For this review, take the finished solid that the model builds, in its own axes (mm). Face numbers are marked on the shaded views. A direction names the side the tool comes from. Round coordinates to 2 decimals unless told otherwise and drop trailing zeros. Write each loop counter-clockwise with the first axis right and the second up, starting at its lowest first coordinate (ties: lowest second). Pieces come first, ordered by that corner, then holes.
from build123d import *

# Parameters (mm, degrees)
SWEEP_THIN1_PROFILE_R   = 10
SWEEP_THIN1_PROFILE_R_2 = 7
SKETCH22_R              = 5
CUT_EXTRUDE1_DEPTH      = 542.256514583
CUT_EXTRUDE1_DEPTH_BACK = 542.256514583


with BuildPart() as part:
    # Sweep-Thin1: sweep along a path in Sketch1
    with BuildLine(Plane(origin=(0, 0, 0), x_dir=(1, 0, 0), z_dir=(0, 1, 0))) as sweep_thin1_path:
        Line((0, 0), (-169.705627485, 169.705627485))
        ThreePointArc((-169.705627485, 169.705627485), (-185.926794926, 180.544265051), (-205.060966544, 184.350288425))
        Line((-205.060966544, 184.350288425), (-505.060966544, 184.350288425))
    # Sweep-Thin1 profile (on start of the path) → Sweep-Thin1 (sweep)
    with BuildSketch(Plane(origin=(0, 0, 0), x_dir=(-0.7071067811865487, 0, 0.7071067811865465), z_dir=(-0.7071067811865465, 0, -0.7071067811865487))):
        Circle(SWEEP_THIN1_PROFILE_R)
        Circle(SWEEP_THIN1_PROFILE_R_2, mode=Mode.SUBTRACT)
    sweep(path=sweep_thin1_path.line)

    # Sketch22 → Cut-Extrude1 (cut, two sides)
    with BuildSketch(Plane(origin=(0, 0, 0), x_dir=(1, 0, 0), z_dir=(0, 1, 0))) as cut_extrude1_sk:
        with Locations(Location((-35.355339059, 35.355339059, 0), (0, 0, 270))):
            Circle(SKETCH22_R)
    extrude(amount=CUT_EXTRUDE1_DEPTH, mode=Mode.SUBTRACT)
    extrude(cut_extrude1_sk.sketch, amount=-CUT_EXTRUDE1_DEPTH_BACK, mode=Mode.SUBTRACT)


solid = part.part
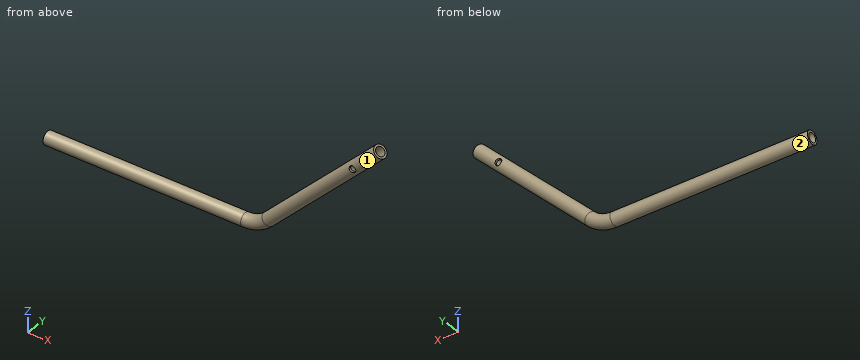
(1) For line 1 along Z through (x, y) = (-387, 1); line 2 along X through (y, z) = (3, -154.5); line 3 along X through (y, z) = (-4, -110), list the stretches that pass through material, from the lowest coordinate up.
Geometry check:
line 1: z = -194.3 to -191.28, -177.42 to -174.4
line 2: x = -167.99 to -163.44, -145.56 to -141.01
line 3: x = -122.96 to -118.12, -101.88 to -97.04
(2) For the marked faces 1 and 2, list the 3-axis set-ups (+Z, -Z, +X, -X, +Y, -Y) from which the entire face can be reached by the end or side of a thin tool; tool diameter is ignored.
Geometry check:
face 1: none
face 2: -X
(3) We need section B-B, the plane x = -307.5. Give the boundary of the cut face in (y, z).
Geometry check:
outline: circle Ø20 at (0, -184.35); hole circle Ø14 at (0, -184.35)
(4) For pin 1 Ø16 at (x, z) = (-35.36, -35.36) entering from +Y; pin 2 Ø2 at (x, y) = (-58, -1) entering from -Z; pin 3 Ø1.5 at (y, z) = (8, -102.5) entering from +X; pin 4 Ø5 at (x, z) = (-156.5, -173) entering from -Y, all flat-tipped, find the tip position at first contact; note any pin that passes through.
Geometry check:
pin 1: stops at y = 10
pin 2: stops at z = -73.08
pin 3: stops at x = -92.53
pin 4: stops at y = -4
(5) We need section A-A, the plane y = 0. Give the boundary of the cut face in (x, z).
Geometry check:
outline: (-505.06, -194.35) - (-205.06, -194.35) arc R60 ccw to (-162.63, -176.78) - (7.07, -7.07) - (4.95, -4.95) - (-164.76, -174.66) arc R57 cw to (-205.06, -191.35) - (-505.06, -191.35) - close; (-505.06, -177.35) - (-205.06, -177.35) arc R43 ccw to (-174.66, -164.76) - (-4.95, 4.95) - (-7.07, 7.07) - (-176.78, -162.63) arc R40 cw to (-205.06, -174.35) - (-505.06, -174.35) - close
